Autodesk Inventor part; units mm, degrees
ref_plane "Work Plane1" through (0, 0, 0) normal (1, 0, 0) x (0, 1, 0)
ref_plane "Work Plane2" through (0, 0, 0) normal (0.9510565, 0.309017, 0) x (0, 0, 1)
ref_plane "Work Plane3" through (0, 0, 2.3813) normal (0, 0, -1) x (-1, 0, 0)
sketch "Sketch1" plane through (0, 0, 0) normal (0, 0, 1) x (1, 0, 0)
  circle A0 centre (0, 0) radius 24.0825
  dimension "d0" = 48.1651
extrude "Extrusion1" add sketch "Sketch1" along normal blind 4.7625
sketch "Sketch2" plane through (0, 0, 0) normal (0, 0, -1) x (-1, 0, 0)
  circle A0 centre (0, 0) radius 24.0825
  circle A1 centre (0, 0) radius 20
  dimension "d3" = 40
surface extrude "Pitch Diameter" sketch "Sketch2" against normal through all shown no curves A1
ref_plane "Work Plane1" through (0, 0, 0) normal (1, 0, 0) x (0, 1, 0)
ref_plane "Work Plane2" through (0, 0, 0) normal (0.9510565, 0.309017, 0) x (0, 0, 1)
ref_plane "Work Plane3" through (0, 0, 2.3813) normal (0, 0, -1) x (-1, 0, 0)
spur gear teeth "Spur Gear" teeth 10 pitch diameter 40 tip diameter 48.1651 root diameter 30.1732 face width 4.7625 start plane through (0, 0, 0) normal (0, 0, -1) x (-1, 0, 0)
equation "\"d0\" = da_da"
equation "\"d1\" = da_b"
equation "\"d3\" = da_d"
equation "\"d15\" = da_aw"
equation "\"d19\" = da_aw"
properties part number "DRIVEN,INTAKE" material "Steel"
Source: CAD feature listing. Evaluate the final solid. Frame: model axes, mm. A direction names the side the tool comes from. Give positions to 0.01 mm unless a question says otherwise; leave off trailing zeros. Write each loop counter-clockwise with the first axis right and the second up, starting at its lowest first coordinate (ties: lowest second). Pieces come first, ordered by that corner, then holes. Notation, with made-up numbers: (-0.5, 21) -> (7.5, 21) arc R18 cw to (7.5, 33) -> close; hole circle Ø9 at (-17, -38.5). An arc over 180 degrees is marked (long way). Return JSON: item names as keys, results as strings. Group by question number.
1. Mould query, pull axis Y, two halves, no side actions, for faces 1 (the face through (-14.052, -13.887, 2.348)), 2 (the face through (17.417, 9.054, 2.348)), 3 (the face through (22.91, -7.42, 2.35)), 4 (the face through (22.896, 7.467, 2.348)). Classes: +Y half, -Y half, draft (parallel to the pull), parting line (faces both ways), or undercut.
2. Section D-D, the plane x = 7.5. Output: boundary loops of the cut face in (y, z), then the cut area to 3 significant figures.
3. Section A-A, the plane y = 16.5. Output: boundary loops of the cut face in (x, z), then the cut area to 3 significant figures.
4. Material intervals for line 1 (X direction, y = 16, z = 3.75); line 2 (X direction, y = -19, z = 2.6); line 3 (Y direction, x = 13.5, z = 2.3), sorted ascending. Write a range as from..to.
5. Pin query (flat end, axial travel): pin 1 Ø2 at (y, z) = (2.5, 3.5) entering from -X; pin 2 Ø2 at (x, z) = (14.5, 2) entering from -Y; pin 3 Ø1.5 at (y, z) = (-16.5, 1) entering from +X. Return the tip coordinate at first contact, or that it passes through.
6. Section B-B, the plane x = 20. Output: boundary loops of the cut face in (y, z), then the cut area to 3 significant figures.
7. Section C-C, the plane y = -17. Output: boundary loops of the cut face in (x, z).
8. Access query for faces 5 (the face through (-19.531, -2.975, 2.348)), 6 (the face through (8.87, -17.66, 2.35)), 7 (the face through (13.993, -13.767, 2.348)), 8 (the face through (-12.196, -8.881, 2.348)). Directions: +Z, -Z, +X, -X, +Y, -Y. A direction counts if a zero-diameter tool reaches every point of the face in a straight line with its end or side. Return the directions, or none.
Determined:
{
 "1": {"face 1": "undercut", "face 2": "undercut", "face 3": "-Y half", "face 4": "+Y half"},
 "2": {"outline": "(-16.22, 0) -> (16.22, 0) -> (16.22, 4.76) -> (-16.22, 4.76) -> close", "area": "154 mm2"},
 "3": {"outline": "(-15.12, 0) -> (-7.75, 0) -> (-7.75, 4.76) -> (-15.12, 4.76) -> close; (-3.53, 0) -> (3.53, 0) -> (3.53, 4.76) -> (-3.53, 4.76) -> close; (7.75, 0) -> (15.12, 0) -> (15.12, 4.76) -> (7.75, 4.76) -> close", "area": "104 mm2"},
 "4": {"line 1": "x = -14.94..-7.31, -3.54..3.54, 7.31..14.94", "line 2": "x = -14.8..-10.4, -3.29..3.29, 10.4..14.8", "line 3": "y = -19.94..-12.83, -8.11..8.11, 12.83..19.94"},
 "5": {"pin 1": "stops at x = -20.46", "pin 2": "stops at y = -19.94", "pin 3": "stops at x = 15.36"},
 "6": {"outline": "(-9.27, 0) -> (-3.23, 0) -> (-3.23, 4.76) -> (-9.27, 4.76) -> close; (3.23, 0) -> (9.27, 0) -> (9.27, 4.76) -> (3.23, 4.76) -> close", "area": "57.5 mm2"},
 "7": {"outline": "(-15.28, 0) -> (-8.21, 0) -> (-8.21, 4.76) -> (-15.28, 4.76) -> close; (-3.5, 0) -> (3.5, 0) -> (3.5, 4.76) -> (-3.5, 4.76) -> close; (8.21, 0) -> (15.28, 0) -> (15.28, 4.76) -> (8.21, 4.76) -> close"},
 "8": {"face 5": "+Z, -Z, -X", "face 6": "+Z, -Z, -Y", "face 7": "+Z, -Z, +X", "face 8": "+Z, -Z"}
}
